Geometry check sheet. Reference: the model listing, model coordinates, mm. A direction names the side the tool comes from. Round coordinates to 2 decimals unless told otherwise and drop trailing zeros. Write each loop counter-clockwise with the first axis right and the second up, starting at its lowest first coordinate (ties: lowest second). Pieces come first, ordered by that corner, then holes. Notation, with made-up numbers: M -33,86.25 L -23,86.25 A23 ccw -23,110.25 Z; hole C 80,-30.75 d2. An arc over 180 degrees is marked long. Answer in a Markdown table with one row per item. Add a question column.
from build123d import *

# Parameters (mm, degrees)
SKETCH1_W           = 17
SKETCH1_H           = 25
BOSS_EXTRUDE1_DEPTH = 6
SKETCH2_R           = 2
CUT_EXTRUDE1_DEPTH  = 40.990623901
FILLET2_R           = 2
FILLET1_R           = 2
CUT_EXTRUDE2_START  = -4
SKETCH3_R           = 2.5
CUT_EXTRUDE2_DEPTH  = 36.990623901
FILLET3_R           = 1
CHAMFER1_SIZE       = 0.5
SKETCH4_W           = 8
SKETCH4_H           = 9.5
CUT_EXTRUDE3_DEPTH  = 40.990623901
FILLET4_R           = 1


with BuildPart() as part:
    # Sketch1 → Boss-Extrude1 (new body)
    with BuildSketch(Plane(origin=(0, 0, 0), x_dir=(1, 0, 0), z_dir=(0, 1, 0))):
        Polygon((8.5, -12.5), (-8.5, -12.5), (-33.5, -12.5), (-33.5, -21), (8.5, -21), align=None)
        Rectangle(SKETCH1_W, SKETCH1_H)
    extrude(amount=BOSS_EXTRUDE1_DEPTH)

    # Sketch2 → Cut-Extrude1 (cut, through all)
    with BuildSketch(Plane(origin=(0, 6, 0), x_dir=(1, 0, 0), z_dir=(0, 1, 0))):
        with Locations(Location((-2.5, 8.5, 0), (0, 0, 270))):
            Circle(SKETCH2_R)
        with Locations(Location((5.5, -3.5, 0), (0, 0, 270))):
            Circle(SKETCH2_R)
    extrude(amount=-CUT_EXTRUDE1_DEPTH, mode=Mode.SUBTRACT)

    # Fillet2
    fillet2_edges = [part.edges().sort_by_distance(p)[0] for p in [
        (8.5, 3, 21),
        (-33.5, 3, 21),
        (-12.5, 6, 21),
        (-12.5, 0, 21),
    ]]
    fillet(fillet2_edges, radius=FILLET2_R)

    # Fillet1
    fillet1_edges = [part.edges().sort_by_distance(p)[0] for p in [
        (-8.5, 3, 12.5),
        (-8.5, 3, -12.5),
        (8.5, 3, -12.5),
        (-33.5, 3, 12.5),
    ]]
    fillet(fillet1_edges, radius=FILLET1_R)

    # Sketch3 → Cut-Extrude2 (cut, through all)
    with BuildSketch(Plane.XZ.offset(CUT_EXTRUDE2_START)):
        with Locations(Location((5.5, 3.5, 0), (0, 0, 270))):
            Circle(SKETCH3_R)
        with Locations(Location((-2.5, -8.5, 0), (0, 0, 270))):
            Circle(SKETCH3_R)
    extrude(amount=-CUT_EXTRUDE2_DEPTH, mode=Mode.SUBTRACT)

    # Fillet3
    # the kernel refuses this fillet: 1 mm, written as the material it adds along each edge
    with BuildSketch(Plane(origin=(5.5, 4, 3.5), x_dir=(0, 0, -1), z_dir=(-1, 0, 0))) as fillet3_piece_1:
        with BuildLine():
            CenterArc((1.5, -0.866025404), FILLET3_R, 0, 60)
            Line((2.5, -0.866025404), (2.52, -0.866025404))
            Line((2.52, -0.866025404), (2.52, 0))
            Line((2.52, 0), (2.5, 0.02))
            ThreePointArc((2.5, 0.02), (2.25, 0.02), (2.01, 0.017320508))
            Line((2.01, 0.017320508), (2, 0))
        make_face()
    revolve(axis=Axis((5.5, 4, 3.5), (0, -1, 0)))
    with BuildSketch(Plane(origin=(-2.5, 4, -8.5), x_dir=(0, 0, -1), z_dir=(-1, 0, 0))) as fillet3_piece_2:
        with BuildLine():
            CenterArc((1.5, -0.866025404), FILLET3_R, 0, 60)
            Line((2.5, -0.866025404), (2.52, -0.866025404))
            Line((2.52, -0.866025404), (2.52, 0))
            Line((2.52, 0), (2.5, 0.02))
            ThreePointArc((2.5, 0.02), (2.25, 0.02), (2.01, 0.017320508))
            Line((2.01, 0.017320508), (2, 0))
        make_face()
    revolve(axis=Axis((-2.5, 4, -8.5), (0, -1, 0)))

    # Chamfer1
    chamfer1_edges = [part.edges().sort_by_distance(p)[0] for p in [
        (-2.5, 0, -10.5),
        (5.5, 0, 1.5),
    ]]
    chamfer(chamfer1_edges, length=CHAMFER1_SIZE)

    # Sketch4 → Cut-Extrude3 (cut, through all)
    with BuildSketch(Plane(origin=(0, 6, 0), x_dir=(1, 0, 0), z_dir=(0, 1, 0))):
        with Locations((-4.5, -3.5)):
            Rectangle(SKETCH4_W, SKETCH4_H)
    extrude(amount=-CUT_EXTRUDE3_DEPTH, mode=Mode.SUBTRACT)

    # Fillet4
    fillet4_edges = [part.edges().sort_by_distance(p)[0] for p in [
        (-0.5, 3, -1.25),
        (-0.5, 3, 8.25),
        (-8.5, 3, 8.25),
        (-8.5, 3, -1.25),
    ]]
    fillet(fillet4_edges, radius=FILLET4_R)


solid = part.part
Item 1: Scan lines: probe 1 along X at (y, z) = (5.6, -8.5); probe 2 along Z at (x, y) = (-4, 3.4); probe 3 along Z at (x, y) = (5.5, 3.3). Record each from-to range of solid material in increasing order. Write a range as from..to.
Item 2: Section check B-B, the plane z = 3.5. Record the boundary of the cut face in (x, y), and give its area (3 significant figures).
Item 3: Gauge pin test, flat ends, axial feed: pin 1 Ø1 at (y, z) = (1.5, 10) entering from -X; pin 2 Ø2 at (x, z) = (-2.5, 4.5) entering from -Y; pin 3 Ø3 at (x, y) = (-22, 3.5) entering from -Z. Record the tip position at first contact, or that the pin passes through.
Item 4: Section check C-C, the plane x = 5.5. Record the boundary of the cut face in (y, z), and give its area (3 significant figures).
Item 5: Mould release check, pull along X, two halves, no side actions. Record for faces 4 (the flat face through (-21, 3, 12.5)), 5 (the cylindrical face through (6.251, 5.425, 1.115)), 6 (the flat face through (8.5, 3, 4)), 7 (the cylindrical face through (-8.215, 2.958, 8.551)): +X half, -X half, draft (parallel to the pull), parting line (faces both ways), or undercut.
Item 6: Section check D-D, the plane y = 2.5. Record the boundary of the cut face in (x, z), and give its area (3 significant figures).
Item 7: Section check A-A, the plane x = -2.5. Record the boundary of the cut face in (y, z), and give its area (3 significant figures).
Item 8: Access from +Z, -Z, +X, -X, +Y, -Y to the whole of each face (thin tool, end or side, straight path). Record for faces 1 (the cylindrical face through (-0.801, 2.958, 7.965)), 2 (the flat face through (-8.5, 3, -6)), 3 (the cylindrical face through (-12.21, 5.43, 20.4)).
Result sheet:
| question | item | result |
|---|---|---|
| 1 | probe 1 | x = -8.5..-5, 0..8.5 |
| 1 | probe 2 | z = -12.5..-9.82, -7.18..-1.25, 8.25..21 |
| 1 | probe 3 | z = -12.5..1.5, 5.5..21 |
| 2 | outline | M -0.5,0 L 3,0 L 3.5,0.5 L 3.5,4 A1 cw 3,4.87 L 3,6 L -0.5,6 Z; M 7.5,0.5 L 8,0 L 8.5,0 L 8.5,6 L 8,6 L 8,4.87 A1 cw 7.5,4 Z |
| 2 | area | 28.0 mm^2 |
| 3 | pin 1 | stops at x = -8.5 |
| 3 | pin 2 | passes through |
| 3 | pin 3 | stops at z = 12.5 |
| 4 | outline | M 0,-12.5 L 6,-12.5 L 6,1 L 4.87,1 A1 cw 4,1.5 L 0.5,1.5 L 0,1 Z; M 0,6 L 0.5,5.5 L 4,5.5 A1 cw 4.87,6 L 6,6 L 6,19 A2 ccw 4,21 L 2,21 A2 ccw 0,19 Z |
| 4 | area | 173 mm^2 |
| 5 | face 4 | draft |
| 5 | face 5 | undercut |
| 5 | face 6 | +X half |
| 5 | face 7 | -X half |
| 6 | outline | M -33.5,14.5 A2 ccw -31.5,12.5 L -10.5,12.5 A2 cw -8.5,10.5 L -8.5,9.25 A1 ccw -7.5,8.25 L -1.5,8.25 A1 cw -0.5,7.25 L -0.5,-0.25 A1 cw -1.5,-1.25 L -7.5,-1.25 A1 ccw -8.5,-2.25 L -8.5,-10.5 A2 ccw -6.5,-12.5 L 6.5,-12.5 A2 ccw 8.5,-10.5 L 8.5,19 A2 ccw 6.5,21 L -31.5,21 A2 ccw -33.5,19 Z; hole C -2.5,-8.5 d4; hole C 5.5,3.5 d4 |
| 6 | area | 677 mm^2 |
| 7 | outline | M 0,-12.5 L 6,-12.5 L 6,-11 L 4.87,-11 A1 cw 4,-10.5 L 0.5,-10.5 L 0,-11 Z; M 0,-6 L 0.5,-6.5 L 4,-6.5 A1 cw 4.87,-6 L 6,-6 L 6,-1.25 L 0,-1.25 Z; M 0,8.25 L 6,8.25 L 6,19 A2 ccw 4,21 L 2,21 A2 ccw 0,19 Z |
| 7 | area | 116 mm^2 |
| 8 | face 1 | -X, +Y, -Y |
| 8 | face 2 | -Z, -X, +Y, -Y |
| 8 | face 3 | +Z, +X, -X, +Y |
